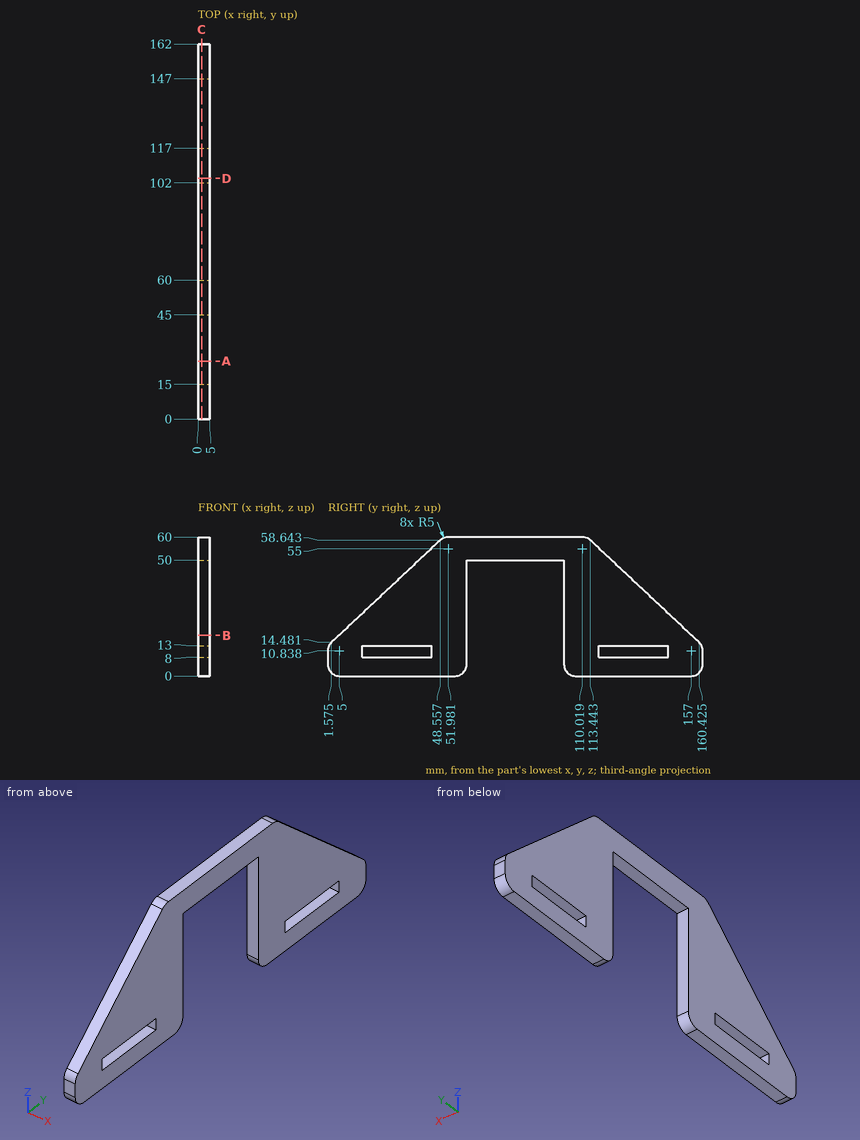
Study the drawing (mm; zero at the part's minimum x, y, z) and answer. Give positions to 0.01 mm unless a question says otherwise; leave off trailing zeros. Order: outer loops, then holes, each group sorted by start corner. A loop starts at its lowest first (then second) coordinate and runs counter-clockwise, first axis right, second up. Notation, with made-up numbers: (-38, -2) - (13, -2) arc R6 cw to (13, 9) - close; hole circle Ø1 at (-34, 8.25). An arc over 180 degrees is marked (long way). Answer in a Markdown table with one row per item. Add a question column.
Q1. The part is cut by section A-A (y = 25). Determine the outline of the cut face in (x, z).
Q2. The part is cut by section C-C (x = 1.5). Determine the outline of the cut face in (y, z) (1 decimal).
Q3. The part is cut by section B-B (z = 17.5). Determine the outline of the cut face in (x, y).
Q4. The part is cut by section D-D (y = 104). Determine the outline of the cut face in (x, z), then the cut area to 3 significant figures.
Q5. Given P1, Ø3, axis at y = 121, z = 10, coming from the +X side; P2, Ø2.5, axis at x = 3, y = 136, coming from the +Z side (1 decimal); P3, Ø3, axis at x = 3, z = 33.5, coming from the -Y side; P4, Ø2, axis at x = 3.5, y = 125, coming from the +Z side, each flat-ended and moving along its own axis, determine where each tip first touches the part or whether it passes through.
Q6. Find the intervals of material crossed by line 1 along Y through (x, z) = (0.85, 11); line 2 along Y through (x, z) = (4.65, 6.5); line 3 along Z through (x, y) = (3.6, 100.5), in increasing order. Write a range as [from, to].
Determined:
| question | item | result |
|---|---|---|
| 1 | outline | (0, 0) - (5, 0) - (5, 8) - (0, 8) - close; (0, 13) - (5, 13) - (5, 36.5) - (0, 36.5) - close |
| 2 | outline | (0, 5) arc R5 ccw to (5, 0) - (55, 0) arc R5 ccw to (60, 5) - (60, 50) - (102, 50) - (102, 5) arc R5 ccw to (107, 0) - (157, 0) arc R5 ccw to (162, 5) - (162, 10.8) arc R5 ccw to (160.4, 14.5) - (113.4, 58.6) arc R5 ccw to (110, 60) - (52, 60) arc R5 ccw to (48.6, 58.6) - (1.6, 14.5) arc R5 ccw to (0, 10.8) - close; hole (15, 8) - (45, 8) - (45, 13) - (15, 13) - close; hole (117, 8) - (147, 8) - (147, 13) - (117, 13) - close |
| 3 | outline | (0, 4.79) - (5, 4.79) - (5, 60) - (0, 60) - close; (0, 102) - (5, 102) - (5, 157.21) - (0, 157.21) - close |
| 4 | outline | (0, 1) - (5, 1) - (5, 60) - (0, 60) - close |
| 4 | area | 295 mm² |
| 5 | P1 | passes through |
| 5 | P2 | stops at z = 38.6 |
| 5 | P3 | stops at y = 20.21 |
| 5 | P4 | stops at z = 48.72 |
| 6 | line 1 | y = [0, 15], [45, 60], [102, 117], [147, 162] |
| 6 | line 2 | y = [0, 60], [102, 162] |
| 6 | line 3 | z = [50, 60] |
